Autodesk Inventor part; units mm, degrees
ref_plane "YZ Plane" through (0, 0, 0) normal (1, 0, 0) x (0, 1, 0)
ref_plane "XZ Plane" through (0, 0, 0) normal (0, 1, 0) x (-1, 0, 0)
ref_plane "XY Plane" through (0, 0, 0) normal (0, 0, 1) x (1, 0, 0)
sketch "Sketch1" plane through (0, 0, 0) normal (0, 1, 0) x (-1, 0, 0)
  line L0 (0, 0) -> (7.7978, 0)
  line L1 (7.7978, 0) -> (7.7978, -15.5956)
  line L2 (7.7978, -15.5956) -> (0, -15.5956)
  line L3 (0, -15.5956) -> (0, 0)
  dimension "d0" = 7.7978
  dimension "d8" = 15.5956
extrude "Extrusion1" add sketch "Sketch1" along normal blind 9.6088
sketch "Sketch2" plane through (0, 9.6088, 0) normal (0, 1, 0) x (1, 0, 0)
  line L0 (-7.7978, 0) -> (0, 0) construction
  line L1 (0, 0) -> (-3.8989, 0) construction
  line L2 (-3.8989, 0) -> (-3.8989, 3.8989) construction
  line L3 (-3.8989, 3.8989) -> (0, 3.8989) construction
  line L4 (0, 3.8989) -> (0, 0) construction
  circle A0 centre (-3.8989, 3.8989) radius 2.4498
  dimension "d11" = 3.8989
  dimension "d12" = 3.8989
  dimension "d13" = 4.8997
extrude "Extrusion2" add sketch "Sketch2" along normal blind 1.9837
pattern_linear "Rectangular Pattern1" count 2 spacing 7.7978 along (0, 0, -1) of "Extrusion2"
shell "Shell1" thickness 1.4732 removed faces 1 at (-2.5993, 0, -5.1985)
sketch "Sketch3" plane through (-6.3246, 8.1356, -1.4732) normal (0, -1, 0) x (1, 0, 0)
  circle A0 centre (2.4257, -2.4257) radius 2.4498 construction
  circle A1 centre (2.4257, -10.2235) radius 2.4498 construction
  line L0 (2.4257, -2.4257) -> (2.4257, -10.2235) construction
  circle A2 centre (2.4257, -6.3246) radius 1.4491
  point P0 (6.3246, 1.4732)
extrude "Extrusion3" add sketch "Sketch3" along normal up to surface (8.1356 mm away)
equation "\"d0\" = d1"
equation "\"d8\" = 2 * d1"
equation "\"d9\" = d3"
equation "\"d11\" = 0.5 * d1"
equation "\"d12\" = 0.5 * d1"
equation "\"d13\" = d4"
equation "\"d14\" = d5"
equation "\"d18\" = d1"
equation "\"d19\" = d6"
equation "\"d20\" = d5"
equation "\"d1\" = 7.7978"
equation "\"d2\" = 3.23596"
equation "\"d3\" = 9.60882"
equation "\"d4\" = 4.89966"
equation "\"d5\" = 1.98374"
equation "\"d6\" = 1.4732"
equation "\"d7\" = 1.23952"
properties part number "1x2 tall white pegged" material "ABS Plastic"
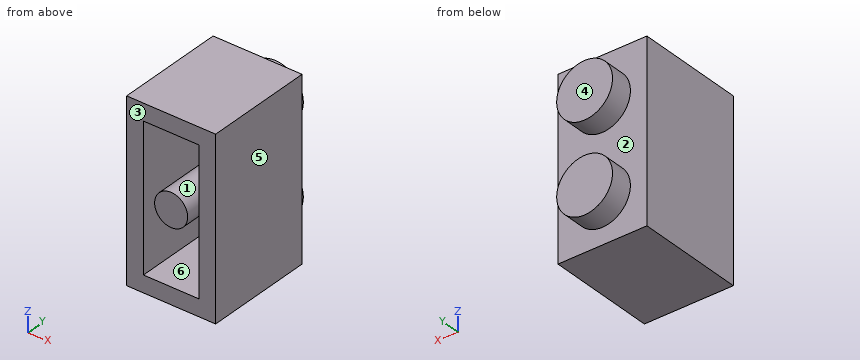
Part model, mm, in its own coordinate system. Face numbers are marked on the shaded views. A direction names the side the tool comes from. Give positions to 0.01 mm unless a question says otherwise; leave off trailing zeros. Write each loop counter-clockwise with the first axis right and the second up, starting at its lowest first coordinate (ties: lowest second). Pieces come first, ordered by that corner, then holes. Notation, with made-up numbers: (68, 28.25) -> (98, 28.25) arc R23 cw to (98, 36.25) -> close; hole circle Ø6 at (-38.75, -11.5). An arc over 180 degrees is marked (long way). Put each result on its own line as item: value. Start each with the question number.
Item 1: Cut at C-C (x = -5.75). List the corners of the cut face in (y, z), then the cut area to 3 significant figures.
Item 2: Cut at A-A (y = 4). List the corners of the cut face in (x, z).
Item 3: Wall check: L1, parallel to X at y = 3, z = -7.75; L2, parallel to X at y = 5.5, z = -3.5; L3, parallel to Z at x = -5.75, y = 1. Give the ranges that are in metal, low to high. Write a range as [from, to].
Item 4: Which spindle directions (+Z, -Z, +X, -X, +Y, -Y) get a long thin tool onto all of the face, cutting with end or side? Do the marked faces 1, 2 and 3. Say none if no direction does.
Item 5: Pin check, flat tips, straight feed: pin 1 Ø1.6 at (x, z) = (-3.5, -4) entering from -Y; pin 2 Ø1.6 at (x, z) = (-3.9, -3.9) entering from -Y. Stop position of each tip, or through.
Item 6: Pull direction X, two halves, no side cores. Call the marked faces 4, 5 and 6: pulls with the +X half, pulls with the -X half, needs draft (parallel to the pull), parting line crosses it, or undercut.
Item 7: Cut at B-B (z = -13). List the corners of the cut face in (x, y).
Item 8: Cut at D-D (z = -11). List the corners of the cut face in (x, y), then the cut area to 3 significant figures.
Answer list:
1. outline: (0, -15.6) -> (9.61, -15.6) -> (9.61, -13.3) -> (11.59, -13.3) -> (11.59, -10.09) -> (9.61, -10.09) -> (9.61, -5.5) -> (11.59, -5.5) -> (11.59, -2.29) -> (9.61, -2.29) -> (9.61, 0) -> (0, 0) -> (0, -1.47) -> (8.14, -1.47) -> (8.14, -14.12) -> (0, -14.12) -> close
1. area: 59.7 mm2
2. outline: (-7.8, -15.6) -> (0, -15.6) -> (0, 0) -> (-7.8, 0) -> close; circle Ø2.9 at (-3.9, -7.8); hole (-6.32, -14.12) -> (-1.47, -14.12) -> (-1.47, -1.47) -> (-6.32, -1.47) -> close
3. L1: x = [-7.8, -6.32], [-5.35, -2.45], [-1.47, 0]
3. L2: x = [-7.8, -6.32], [-1.47, 0]
3. L3: z = [-15.6, -14.12], [-1.47, 0]
4. face 1: -Y
4. face 2: +Y
4. face 3: +Z, -Z, +X, -X, -Y
5. pin 1: stops at y = 8.14
5. pin 2: stops at y = 10.12
6. face 4: needs draft
6. face 5: pulls with the +X half
6. face 6: undercut
7. outline: (-7.8, 0) -> (-6.32, 0) -> (-6.32, 8.14) -> (-1.47, 8.14) -> (-1.47, 0) -> (0, 0) -> (0, 9.61) -> (-1.82, 9.61) -> (-1.82, 11.59) -> (-5.97, 11.59) -> (-5.97, 9.61) -> (-7.8, 9.61) -> close
8. outline: (-7.8, 0) -> (-6.32, 0) -> (-6.32, 8.14) -> (-4.58, 8.14) -> (-4.58, 10.12) -> (-3.21, 10.12) -> (-3.21, 8.14) -> (-1.47, 8.14) -> (-1.47, 0) -> (0, 0) -> (0, 9.61) -> (-1.55, 9.61) -> (-1.55, 11.59) -> (-6.25, 11.59) -> (-6.25, 9.61) -> (-7.8, 9.61) -> close
8. area: 42.1 mm2
